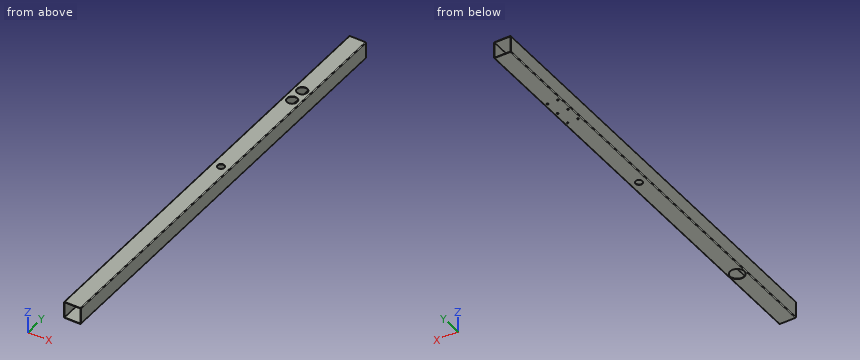
```python
from build123d import *

# Parameters (mm, degrees)
SKETCH1_W           = 65
SKETCH1_H           = 65
SKETCH1_W_2         = 61
SKETCH1_H_2         = 61
BOSS_EXTRUDE1_DEPTH = 1700
CUT_EXTRUDE1_REACH  = 1703.553
SKETCH2_R           = 3
SKETCH2_R_2         = 27.5
FILLET1_R           = 3
CUT_EXTRUDE2_REACH  = 1703.553
SKETCH3_R           = 20
SKETCH4_R           = 13.5
CUT_EXTRUDE3_DEPTH  = 1702.552599833


with BuildPart() as part:
    # Sketch1 → Boss-Extrude1 (new body)
    with BuildSketch(Plane(origin=(0, 0, 0), x_dir=(1, 0, 0), z_dir=(0, 1, 0))):
        Rectangle(SKETCH1_W, SKETCH1_H)
        Rectangle(SKETCH1_W_2, SKETCH1_H_2, mode=Mode.SUBTRACT)
    extrude(amount=BOSS_EXTRUDE1_DEPTH)

    # Sketch2 → Cut-Extrude1 (cut, up to next)
    with BuildSketch(Plane(origin=(0, 0, -32.5), x_dir=(-1, 0, 0), z_dir=(0, 0, -1)), mode=Mode.PRIVATE) as cut_extrude1_sk1:
        with Locations((20, 1400)):
            Circle(SKETCH2_R)
    cut_extrude1_tool1 = extrude(cut_extrude1_sk1.sketch, amount=-CUT_EXTRUDE1_REACH, mode=Mode.PRIVATE) & part.part
    # Sketch2 → Cut-Extrude1 (cut, up to next)
    with BuildSketch(Plane(origin=(0, 0, -32.5), x_dir=(-1, 0, 0), z_dir=(0, 0, -1)), mode=Mode.PRIVATE) as cut_extrude1_sk2:
        with Locations((-20, 1400)):
            Circle(SKETCH2_R)
    cut_extrude1_tool2 = extrude(cut_extrude1_sk2.sketch, amount=-CUT_EXTRUDE1_REACH, mode=Mode.PRIVATE) & part.part
    # Sketch2 → Cut-Extrude1 (cut, up to next)
    with BuildSketch(Plane(origin=(0, 0, -32.5), x_dir=(-1, 0, 0), z_dir=(0, 0, -1)), mode=Mode.PRIVATE) as cut_extrude1_sk3:
        with Locations((20, 1340)):
            Circle(SKETCH2_R)
    cut_extrude1_tool3 = extrude(cut_extrude1_sk3.sketch, amount=-CUT_EXTRUDE1_REACH, mode=Mode.PRIVATE) & part.part
    # Sketch2 → Cut-Extrude1 (cut, up to next)
    with BuildSketch(Plane(origin=(0, 0, -32.5), x_dir=(-1, 0, 0), z_dir=(0, 0, -1)), mode=Mode.PRIVATE) as cut_extrude1_sk4:
        with Locations((-20, 1340)):
            Circle(SKETCH2_R)
    cut_extrude1_tool4 = extrude(cut_extrude1_sk4.sketch, amount=-CUT_EXTRUDE1_REACH, mode=Mode.PRIVATE) & part.part
    # Sketch2 → Cut-Extrude1 (cut, up to next)
    with BuildSketch(Plane(origin=(0, 0, -32.5), x_dir=(-1, 0, 0), z_dir=(0, 0, -1)), mode=Mode.PRIVATE) as cut_extrude1_sk5:
        with Locations(Location((-20, 1280, 0), (0, 0, 180))):
            Circle(SKETCH2_R)
    cut_extrude1_tool5 = extrude(cut_extrude1_sk5.sketch, amount=-CUT_EXTRUDE1_REACH, mode=Mode.PRIVATE) & part.part
    # Sketch2 → Cut-Extrude1 (cut, up to next)
    with BuildSketch(Plane(origin=(0, 0, -32.5), x_dir=(-1, 0, 0), z_dir=(0, 0, -1)), mode=Mode.PRIVATE) as cut_extrude1_sk6:
        with Locations(Location((20, 1280, 0), (0, 0, 180))):
            Circle(SKETCH2_R)
    cut_extrude1_tool6 = extrude(cut_extrude1_sk6.sketch, amount=-CUT_EXTRUDE1_REACH, mode=Mode.PRIVATE) & part.part
    # Sketch2 → Cut-Extrude1 (cut, up to next)
    with BuildSketch(Plane(origin=(0, 0, -32.5), x_dir=(-1, 0, 0), z_dir=(0, 0, -1)), mode=Mode.PRIVATE) as cut_extrude1_sk7:
        with Locations((0, 300)):
            Circle(SKETCH2_R_2)
    cut_extrude1_tool7 = extrude(cut_extrude1_sk7.sketch, amount=-CUT_EXTRUDE1_REACH, mode=Mode.PRIVATE) & part.part
    add(cut_extrude1_tool1.solids().sort_by_distance((-20, 1400, -32.5))[0], mode=Mode.SUBTRACT)
    add(cut_extrude1_tool2.solids().sort_by_distance((20, 1400, -32.5))[0], mode=Mode.SUBTRACT)
    add(cut_extrude1_tool3.solids().sort_by_distance((-20, 1340, -32.5))[0], mode=Mode.SUBTRACT)
    add(cut_extrude1_tool4.solids().sort_by_distance((20, 1340, -32.5))[0], mode=Mode.SUBTRACT)
    add(cut_extrude1_tool5.solids().sort_by_distance((20, 1280, -32.5))[0], mode=Mode.SUBTRACT)
    add(cut_extrude1_tool6.solids().sort_by_distance((-20, 1280, -32.5))[0], mode=Mode.SUBTRACT)
    add(cut_extrude1_tool7.solids().sort_by_distance((0, 300, -32.5))[0], mode=Mode.SUBTRACT)

    # Fillet1
    fillet1_edges = [part.edges().sort_by_distance(p)[0] for p in [
        (32.5, 850, 32.5),
        (-32.5, 850, 32.5),
        (-32.5, 850, -32.5),
        (32.5, 850, -32.5),
    ]]
    fillet(fillet1_edges, radius=FILLET1_R)

    # Sketch3 → Cut-Extrude2 (cut, up to next)
    with BuildSketch(Plane.XY.offset(32.5), mode=Mode.PRIVATE) as cut_extrude2_sk1:
        with Locations((0, 1370)):
            Circle(SKETCH3_R)
    cut_extrude2_tool1 = extrude(cut_extrude2_sk1.sketch, amount=-CUT_EXTRUDE2_REACH, mode=Mode.PRIVATE) & part.part
    # Sketch3 → Cut-Extrude2 (cut, up to next)
    with BuildSketch(Plane.XY.offset(32.5), mode=Mode.PRIVATE) as cut_extrude2_sk2:
        with Locations((0, 1310)):
            Circle(SKETCH3_R)
    cut_extrude2_tool2 = extrude(cut_extrude2_sk2.sketch, amount=-CUT_EXTRUDE2_REACH, mode=Mode.PRIVATE) & part.part
    add(cut_extrude2_tool1.solids().sort_by_distance((0, 1370, 32.5))[0], mode=Mode.SUBTRACT)
    add(cut_extrude2_tool2.solids().sort_by_distance((0, 1310, 32.5))[0], mode=Mode.SUBTRACT)

    # Sketch4 → Cut-Extrude3 (cut, through all)
    with BuildSketch(Plane(origin=(0, 0, -32.5), x_dir=(-1, 0, 0), z_dir=(0, 0, -1))):
        with Locations((0, 885.5)):
            Circle(SKETCH4_R)
    extrude(amount=-CUT_EXTRUDE3_DEPTH, mode=Mode.SUBTRACT)


solid = part.part
```
Work out the finished part from the listing and answer in its coordinate system (mm). Round coordinates to 2 decimals unless told otherwise and drop trailing zeros. Order: outer loops, then holes, each group sorted by start corner. A loop starts at its lowest first (then second) coordinate and runs counter-clockwise, first axis right, second up.
Q1. A cutting plane is placed at A-A, the plane z = 17.5. Determine the outline of the cut face in (x, y).
Solution:
outline: (-32.5, 0) - (-30.5, 0) - (-30.5, 1700) - (-32.5, 1700) - close; (30.5, 0) - (32.5, 0) - (32.5, 1700) - (30.5, 1700) - close
Q2. A cutting plane is placed at C-C, the plane y = 1548. Determine the outline of the cut face in (x, z), then the cut area to 3 significant figures.
Solution:
outline: (-32.5, -29.5) arc R3 ccw to (-29.5, -32.5) - (29.5, -32.5) arc R3 ccw to (32.5, -29.5) - (32.5, 29.5) arc R3 ccw to (29.5, 32.5) - (-29.5, 32.5) arc R3 ccw to (-32.5, 29.5) - close; hole (-30.5, -30.5) - (30.5, -30.5) - (30.5, 30.5) - (-30.5, 30.5) - close
area: 496 mm2
Q3. A cutting plane is placed at B-B, the plane y = 1310. Determine the outline of the cut face in (x, z).
Solution:
outline: (-32.5, -29.5) arc R3 ccw to (-29.5, -32.5) - (29.5, -32.5) arc R3 ccw to (32.5, -29.5) - (32.5, 29.5) arc R3 ccw to (29.5, 32.5) - (20, 32.5) - (20, 30.5) - (30.5, 30.5) - (30.5, -30.5) - (-30.5, -30.5) - (-30.5, 30.5) - (-20, 30.5) - (-20, 32.5) - (-29.5, 32.5) arc R3 ccw to (-32.5, 29.5) - close
Q4. A cutting plane is placed at D-D, the plane x = 1. Determine the outline of the cut face in (y, z).
Solution:
outline: (0, -32.5) - (272.52, -32.5) - (272.52, -30.5) - (0, -30.5) - close; (0, 30.5) - (872.04, 30.5) - (872.04, 32.5) - (0, 32.5) - close; (327.48, -32.5) - (872.04, -32.5) - (872.04, -30.5) - (327.48, -30.5) - close; (898.96, -32.5) - (1700, -32.5) - (1700, -30.5) - (898.96, -30.5) - close; (898.96, 30.5) - (1290.03, 30.5) - (1290.03, 32.5) - (898.96, 32.5) - close; (1329.97, 30.5) - (1350.03, 30.5) - (1350.03, 32.5) - (1329.97, 32.5) - close; (1389.97, 30.5) - (1700, 30.5) - (1700, 32.5) - (1389.97, 32.5) - close
Q5. Find the intervals of material crossed by line 1 along X through (y, z) = (1550.5, -19.5); line 2 along Y through (x, z) = (0, 31), in increasing order.
Solution:
line 1: x = -32.5 to -30.5, 30.5 to 32.5
line 2: y = 0 to 872, 899 to 1290, 1330 to 1350, 1390 to 1700
Q6. Given pin 1 Ø3.5 at (x, y) = (20, 1340) entering from -Z, flat-ended and moving along its own axis, determine where the tip first touches the part or whether it passes through.
Solution:
pin 1: stops at z = 30.5
